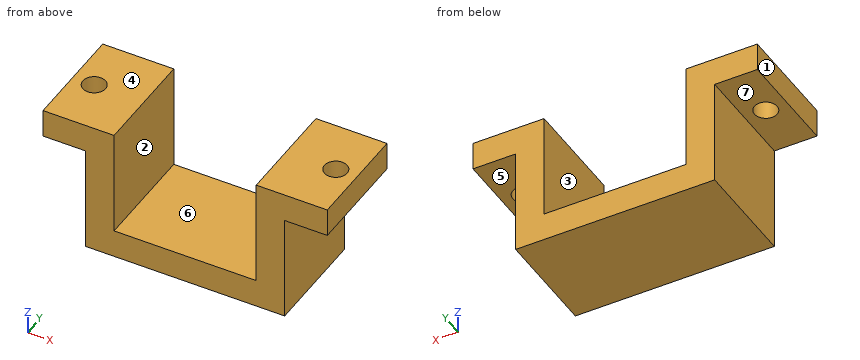
from build123d import *

# Parameters (mm, degrees)
BOSS_EXTRUDE1_DEPTH = 9.525
CUT_EXTRUDE1_REACH  = 4.54
SKETCH2_R           = 1.016


with BuildPart() as part:
    # Sketch1 → Boss-Extrude1 (new body)
    with BuildSketch(Plane(origin=(0, 0, 0), x_dir=(1, 0, 0), z_dir=(0, 1, 0))):
        Polygon((0, 0), (6.35, 0), (6.35, 9.525), (19.05, 9.525), (19.05, 0), (25.4, 0), (25.4, 2.54), (21.59, 2.54), (21.59, 12.065), (3.81, 12.065), (3.81, 2.54), (0, 2.54), align=None)
    extrude(amount=BOSS_EXTRUDE1_DEPTH)

    # Sketch2 → Cut-Extrude1 (cut, up to next)
    with BuildSketch(Plane(origin=(0, 0, -2.54), x_dir=(-1, 0, 0), z_dir=(0, 0, -1)), mode=Mode.PRIVATE) as cut_extrude1_sk1:
        with Locations((-1.905, 4.7625)):
            Circle(SKETCH2_R)
    cut_extrude1_tool1 = extrude(cut_extrude1_sk1.sketch, amount=-CUT_EXTRUDE1_REACH, mode=Mode.PRIVATE) & part.part
    add(cut_extrude1_tool1.solids().sort_by_distance((1.905, 4.7625, -2.54))[0], mode=Mode.SUBTRACT)
    # Sketch2 → Cut-Extrude1 (cut, up to next)
    with BuildSketch(Plane(origin=(0, 0, -2.54), x_dir=(-1, 0, 0), z_dir=(0, 0, -1)), mode=Mode.PRIVATE) as cut_extrude1_sk2:
        with Locations((-23.495, 4.7625)):
            Circle(SKETCH2_R)
    cut_extrude1_tool2 = extrude(cut_extrude1_sk2.sketch, amount=-CUT_EXTRUDE1_REACH, mode=Mode.PRIVATE) & part.part
    add(cut_extrude1_tool2.solids().sort_by_distance((23.495, 4.7625, -2.54))[0], mode=Mode.SUBTRACT)


solid = part.part
Can you work these out from the model? Positions are in its coordinate system, mm. Face numbers are marked on the shaded views. A direction names the side the tool comes from. Round coordinates to 2 decimals unless told otherwise and drop trailing zeros. Write each loop counter-clockwise with the first axis right and the second up, starting at its lowest first coordinate (ties: lowest second). Pieces come first, ordered by that corner, then holes. Notation, with made-up numbers: (76, 1) -> (109, 1) arc R23 cw to (109, 40) -> close; hole circle Ø7 at (16, 45.5). An arc over 180 degrees is marked (long way). Use one line per item in the form item = value. Start each with the question number.
Q1. I'm going to push flat-ended pins straight in: P1, Ø1.5, axis at y = 3.5, z = -5.5, coming from the -X side; P2, Ø5, axis at x = 9.5, y = 7.5, coming from the +Z side (3 decimals); P3, Ø1.1, axis at x = 24.5, y = 5, coming from the -Z side. Where does each tip first touch, or does it pass through?
Q2. Imagine slicing it at D-D (y = 5.5). Please give me the cut outline in (x, z) (3 decimals), then the cut area to 3 significant figures.
Q3. Imagine slicing it at C-C (y = 1.75). Please give me the cut outline in (x, z) (3 decimals).
Q4. Imagine slicing it at B-B (z = -1). Count the separate pieces of the cut face and the enclosed holes in it, then the cut area to 3 significant figures.
Q5. If I drill on probe 1 along X at (y, z) = (1.25, -3.25); probe 2 along X at (y, z) = (0.5, -2.5); probe 3 along Z at (x, y) = (7.5, 5.5) (3 decimals), over which ranges is the centre line in solid material (lowest first)? Write a range as [from, to].
Q6. Which directions (+Z, -Z, +X, -X, +Y, -Y) give clear straight access to the entire face, cutting with the end or side of a thin tool? Please do the marked faces 5, 6 and 7.
Q7. We'd pull the mould along X, two halves only. Please class the marked faces 1, 2, 3 and 4: +X half, -X half, draft (parallel to the pull), parting line (faces both ways), or undercut.
Q8. Imagine slicing it at A-A (z = -6.5). Please give me the cut outline in (x, y) (3 decimals), then the cut area to 3 significant figures.
Worked out:
q1.P1 = 3.81
q1.P2 = -9.525
q1.P3 = -2.54
q2.outline = (0, -2.54) -> (1.206, -2.54) -> (1.206, 0) -> (0, 0) -> close; (2.604, -2.54) -> (3.81, -2.54) -> (3.81, -12.065) -> (21.59, -12.065) -> (21.59, -2.54) -> (22.796, -2.54) -> (22.796, 0) -> (19.05, 0) -> (19.05, -9.525) -> (6.35, -9.525) -> (6.35, 0) -> (2.604, 0) -> close; (24.194, -2.54) -> (25.4, -2.54) -> (25.4, 0) -> (24.194, 0) -> close
q2.area = 106 mm^2
q3.outline = (0, -2.54) -> (3.81, -2.54) -> (3.81, -12.065) -> (21.59, -12.065) -> (21.59, -2.54) -> (25.4, -2.54) -> (25.4, 0) -> (19.05, 0) -> (19.05, -9.525) -> (6.35, -9.525) -> (6.35, 0) -> (0, 0) -> close
q4.separate_pieces = 2
q4.enclosed_holes = 2
q4.area = 114 mm^2
q5.probe_1 = [3.81, 6.35], [19.05, 21.59]
q5.probe_2 = [0, 6.35], [19.05, 25.4]
q5.probe_3 = [-12.065, -9.525]
q6.face_5 = -Z, +X, +Y, -Y
q6.face_6 = +Z, +Y, -Y
q6.face_7 = -Z, -X, +Y, -Y
q7.face_1 = -X half
q7.face_2 = undercut
q7.face_3 = undercut
q7.face_4 = draft
q8.outline = (3.81, 0) -> (6.35, 0) -> (6.35, 9.525) -> (3.81, 9.525) -> close; (19.05, 0) -> (21.59, 0) -> (21.59, 9.525) -> (19.05, 9.525) -> close
q8.area = 48.4 mm^2
